from build123d import *

# Parameters (mm, degrees)
SKETCH1_R           = 4.25
SKETCH1_W           = 20
SKETCH1_H           = 5
BOSS_EXTRUDE1_DEPTH = 3
SKETCH2_R           = 7
SKETCH2_R_2         = 4.25
BOSS_EXTRUDE2_DEPTH = 1
FILLET1_R           = 1


with BuildPart() as part:
    # Sketch1 → Boss-Extrude1 (new body)
    with BuildSketch(Plane.XY):
        with BuildLine():
            Line((9, -33.5), (-26, -33.5))
            ThreePointArc((-26, -33.5), (-33, -26.5), (-26, -19.5))
            Line((-26, -19.5), (-20, -19.5))
            ThreePointArc((-20, -19.5), (-16.464466094, -18.035533906), (-15, -14.5))
            Line((-15, -14.5), (-15, 28.5))
            ThreePointArc((-15, 28.5), (-13.535533906, 32.035533906), (-10, 33.5))
            Line((-10, 33.5), (10, 33.5))
            ThreePointArc((10, 33.5), (13.535533906, 32.035533906), (15, 28.5))
            Line((15, 28.5), (15, -22.894448725))
            ThreePointArc((15, -22.894448725), (15.092571663, -29.946820352), (9, -33.5))
        make_face()
        with Locations((9, -26.5)):
            Circle(SKETCH1_R, mode=Mode.SUBTRACT)
        with Locations((-26, -26.5)):
            Circle(SKETCH1_R, mode=Mode.SUBTRACT)
        with Locations((0, 26)):
            Rectangle(SKETCH1_W, SKETCH1_H, mode=Mode.SUBTRACT)
    extrude(amount=BOSS_EXTRUDE1_DEPTH)

    # Sketch2 → Boss-Extrude2 (add)
    # profile 1 of 2: a face of its own
    with BuildSketch(Plane.XY.offset(3)):
        with Locations(Location((-26, -26.5, 0), (0, 0, 270))):
            Circle(SKETCH2_R)
        with Locations((-26, -26.5)):
            Circle(SKETCH2_R_2, mode=Mode.SUBTRACT)
    # profile 2 of 2: a face of its own
    with BuildSketch(Plane.XY.offset(3)):
        with Locations(Location((9, -26.5, 0), (0, 0, 270))):
            Circle(SKETCH2_R)
        with Locations((9, -26.5)):
            Circle(SKETCH2_R_2, mode=Mode.SUBTRACT)
    extrude(amount=BOSS_EXTRUDE2_DEPTH)

    # Fillet1
    fillet1_edges = [part.edges().sort_by_distance(p)[0] for p in [
        (-26, -19.5, 4),
        (9, -19.5, 4),
    ]]
    fillet(fillet1_edges, radius=FILLET1_R - 0.0001)  # a hair under: the kernel refuses the full size


solid = part.part
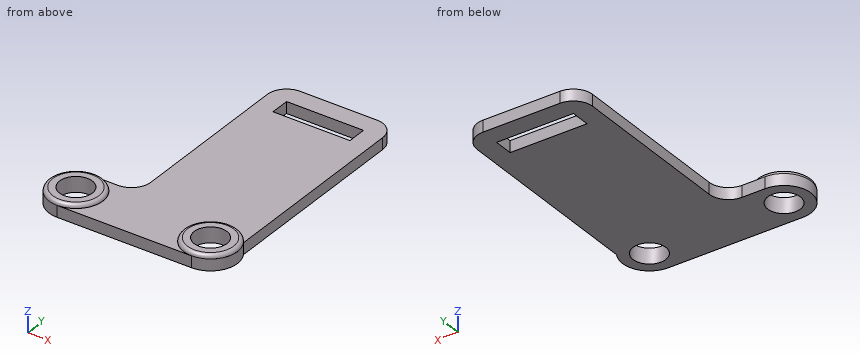
Design review of the part built by this model. Coordinates are the model's own, in mm. Coordinates: 2 decimals unless noted, no trailing zeros. Write each loop counter-clockwise with the first axis right and the second up, starting at its lowest first coordinate (ties: lowest second). Pieces come first, ordered by that corner, then holes. Notation, with made-up numbers: (-20.5, 53) - (-14.5, 53) arc R12 ccw to (-14.5, 67) - close; hole circle Ø8 at (2.5, -22). An arc over 180 degrees is marked (long way). One line per item, written item: value.
1) Add section C-C (z = 0.8). State the section outline as (x, y) points, plus the area to 3 significant figures.
Answer sheet:
outline: (-26, -33.5) - (9, -33.5) arc R7 ccw to (15, -22.89) - (15, 28.5) arc R5 ccw to (10, 33.5) - (-10, 33.5) arc R5 ccw to (-15, 28.5) - (-15, -14.5) arc R5 cw to (-20, -19.5) - (-26, -19.5) arc R7 ccw to start; hole circle Ø8.5 at (-26, -26.5); hole (-10, 23.5) - (10, 23.5) - (10, 28.5) - (-10, 28.5) - close; hole circle Ø8.5 at (9, -26.5)
area: 2,020 mm2
2) Insertion check: pin 1 (2 mm diameter, centred on x = -17, y = 3, fed in from -Z); pin 2 (1.5 mm diameter, centred on x = -23.5, z = 1, fed in from +Y); pin 3 (1.5 mm diameter, centred on y = 6.5, z = 1, fed in from +X); pin 4 (4 mm diameter, centred on x = 1.5, y = 23.5, fed in from +Z). Each pin has a flat end and moves straight along its axis. Give the tip position at first contact, or say it passes through.
Answer sheet:
pin 1: passes through
pin 2: stops at y = -19.5
pin 3: stops at x = 15
pin 4: stops at z = 3
3) Add section A-A (y = 27.5). State the section outline as (x, z) points, plus the area to 3 significant figures.
Answer sheet:
outline: (-15, 0) - (-10, 0) - (-10, 3) - (-15, 3) - close; (10, 0) - (15, 0) - (15, 3) - (10, 3) - close
area: 30.0 mm2
4) To check wall thickness, follow probe 1 along Y at (x, z) = (9, 1.5); probe 2 along Y at (x, z) = (-26, 0.95); probe 3 along Z at (x, y) = (-5, 3). State the ranges of each line that lie inside material, in increasing order.
Answer sheet:
probe 1: y = -33.5 to -30.75, -22.25 to 23.5, 28.5 to 33.5
probe 2: y = -33.5 to -30.75, -22.25 to -19.5
probe 3: z = 0 to 3
5) Add section B-B (x = 1). State the section outline as (y, z) points, plus the area to 3 significant figures.
Answer sheet:
outline: (-33.5, 0) - (23.5, 0) - (23.5, 3) - (-33.5, 3) - close; (28.5, 0) - (33.5, 0) - (33.5, 3) - (28.5, 3) - close
area: 186 mm2
6) Add section D-D (y = -10.5). State the section outline as (x, z) points.
Answer sheet:
outline: (-15, 0) - (15, 0) - (15, 3) - (-15, 3) - close
